Part model, mm, in its own coordinate system. A direction names the side the tool comes from. Give positions to 0.01 mm unless a question says otherwise; leave off trailing zeros. Write each loop counter-clockwise with the first axis right and the second up, starting at its lowest first coordinate (ties: lowest second). Pieces come first, ordered by that corner, then holes.
```python
from build123d import *

# Parameters (mm, degrees)
F0_R     = 1.25
F0_R_2   = 0.5
F1_DEPTH = 5
F2_R     = 2


# Not quite as in the source:
# - two fillets or chamfers of one size are made in one step
# - a feature names something its author has since deleted; it is built from what else it names


with BuildPart() as f1:
    # F0 (on Top) → F1 (new body)
    with BuildSketch(Plane.XY):
        with BuildLine():
            Line((-14.5326076762, 20.3421560836), (-8.1431852604, 12.5971637211))
            ThreePointArc((-8.1431852604, 12.5971637211), (7.1712000772, 13.174744379), (15, 0))
            Line((15, 0), (-2.1995428838, -33.3545495937))
            ThreePointArc((-2.1995428838, -33.3545495937), (-6.9846930225, -40.4626698406), (-1.3037745428, -46.8775120459))
            ThreePointArc((-1.3037745428, -46.8775120459), (1.2316251761, -46.8907981704), (3.6054450158, -46.0000638528))
            Line((3.6054450158, -46.0000638528), (6.9816735201, -39.4938035379))
            Line((6.9816735201, -39.4938035379), (24.1795416276, -6.3521466198))
            ThreePointArc((24.1795416276, -6.3521466198), (14.1919795262, 20.5812467341), (-14.5326076762, 20.3421560836))
        make_face()
        with Locations((0, -40)):
            Circle(F0_R, mode=Mode.SUBTRACT)
        with Locations((4.1248112098, -32.0008792681)):
            Circle(F0_R_2, mode=Mode.SUBTRACT)
        with Locations((13.0337394799, -14.7240660517)):
            Circle(F0_R_2, mode=Mode.SUBTRACT)
        with Locations((15.8593580654, -9.2444300009)):
            Circle(F0_R_2, mode=Mode.SUBTRACT)
        with BuildLine():
            ThreePointArc((3.6054450158, -46.0000638528), (1.2316251761, -46.8907981704), (-1.3037745428, -46.8775120459))
            Line((-1.3037745428, -46.8775120459), (-4.8843406974, -53.3048406851))
            Line((-4.8843406974, -53.3048406851), (-1.2389638203, -55.3356242034))
            Line((-1.2389638203, -55.3356242034), (3.6054450158, -46.0000638528))
        make_face()
        with BuildLine():
            ThreePointArc((3.6054450158, -46.0000638528), (6.2132620695, -43.2241858593), (6.9816735201, -39.4938035379))
            Line((6.9816735201, -39.4938035379), (3.6054450158, -46.0000638528))
        make_face()
    extrude(amount=F1_DEPTH)

    # F2
    f2_edges = [f1.edges().sort_by_distance(p)[0] for p in [
        (6.981674, -39.493804, 2.5),
        (15, 0, 2.5),
        (-8.143185, 12.597164, 2.5),
        (-14.532608, 20.342156, 2.5),
        (24.179542, -6.352147, 2.5),
        (-2.199543, -33.35455, 2.5),
        (-4.884341, -53.304841, 2.5),
        (-1.238964, -55.335624, 2.5),
        (3.605445, -46.000064, 2.5),
    ]]
    fillet(f2_edges, radius=F2_R)


solid = f1.part
```
1) Wall check: L1, parallel to Y at x = -1, z = 3.15; L2, parallel to Y at x = -2.5, z = 0.3; L3, parallel to Y at x = 2, z = 4.8. Give the ranges that are in metal, low to high.
Answers follow:
L1: y = -54.28 to -40.75, -39.25 to -31.03, 14.97 to 24.98
L2: y = -54.54 to -49.02, -46.54 to -33.41, 14.79 to 24.87
L3: y = -49.09 to -25.21, 14.87 to 24.92
2) Saw through at B-B, the plane z = 0.8. Write the cut outline in (x, y), then the cut area to 3 significant figures.
Answers follow:
outline: (-13.1, 18.61) - (-9.22, 13.9) arc R2 ccw to (-6.77, 13.39) arc R15 cw to (14.99, 0.54) arc R2 cw to (14.77, -0.45) - (-1.85, -32.68) arc R2 cw to (-2.82, -33.59) arc R7 ccw to (-1.3, -46.88) - (-3.91, -51.56) arc R2 ccw to (-3.14, -54.28) - (-3.04, -54.33) arc R2 ccw to (-0.29, -53.51) - (3.36, -46.47) arc R2 cw to (4, -45.75) arc R7 ccw to (7, -39.96) arc R2 cw to (7.22, -39.03) - (24.07, -6.55) arc R2 ccw to (24.24, -6.12) arc R25 ccw to (-12.57, 21.61) arc R2 ccw to start; hole circle Ø2.5 at (0, -40); hole circle Ø1 at (4.12, -32); hole circle Ø1 at (13.03, -14.72); hole circle Ø1 at (15.86, -9.24)
area: 1,040 mm2
3) Saw through at A-A, the plane x = -6. Write the cut outline in (y, z).
Answers follow:
outline: (-43.61, 0) - (-36.39, 0) - (-36.39, 5) - (-43.61, 5) - close; (13.75, 0) - (24.27, 0) - (24.27, 5) - (13.75, 5) - close
4) Saw through at C-C, the plane y = -17. Write the cut outline in (x, z).
Answers follow:
outline: (6.23, 0) - (18.65, 0) - (18.65, 5) - (6.23, 5) - close
5) Two-plate mould, pull along Y, no slides. Class faces 4 (the face through (1.51, -50.04, 2.46)), 5 (the face through (0.577, -41.109, 2.465)), 6 (the face through (10, -12, 5)): +Y half, -Y half, draft (parallel to the pull), parting line (faces both ways), or undercut.
Answers follow:
face 4: -Y half
face 5: undercut
face 6: draft
6) 3-axis set-ups, long thin cutter, end or side, ignore diameter. For faces 1 (the face through (7.443, 13.023, 2.465)), 2 (the face through (-11.2, 16.3, 2.5)), 3 (the face through (6.575, -16.339, 2.465)): which of +Z, -Z, +X, -X, +Y, -Y reach the whole face in a straight line?
Answers follow:
face 1: +Z, -Z
face 2: +Z, -Z, -X, -Y
face 3: +Z, -Z, -X
7) Saw through at D-D, the plane x = 22. Write the cut outline in (y, z).
Answers follow:
outline: (-10.55, 0) - (11.87, 0) - (11.87, 5) - (-10.55, 5) - close
8) Pin check, flat tips, straight feed: pin 1 Ø1 at (y, z) = (-4.5, 2) entering from +X; pin 2 Ø1 at (y, z) = (-45.5, 3) entering from +X; pin 3 Ø1 at (x, z) = (8.5, 3) entering from +Y. Stop position of each tip, or through.
Answers follow:
pin 1: stops at x = 24.68
pin 2: stops at x = 4.9
pin 3: stops at y = 23.69
